from build123d import *

# Parameters (mm, degrees)
SKETCH1_W           = 35.56
SKETCH1_H           = 25.08
BOSS_EXTRUDE1_DEPTH = 0.95
SKETCH2_W           = 26.5
SKETCH2_H           = 18
BOSS_EXTRUDE2_DEPTH = 1.5
BOSS_EXTRUDE3_DEPTH = 1.5
SKETCH4_W           = 10
SKETCH4_H           = 3.18
BOSS_EXTRUDE4_DEPTH = 1.56
SKETCH5_R           = 1
SKETCH5_R_2         = 0.875
SKETCH5_R_3         = 0.2
BOSS_EXTRUDE5_DEPTH = 1.5
SKETCH6_W           = 15.5
SKETCH6_H           = 1.85
SKETCH6_W_2         = 15
SKETCH6_H_2         = 1.35
BOSS_EXTRUDE6_DEPTH = 0.75
SKETCH7_R           = 1
CUT_EXTRUDE1_DEPTH  = 3.51
SKETCH8_R           = 1
CUT_EXTRUDE2_DEPTH  = 3.45
SKETCH9_R           = 1.7
SKETCH9_R_2         = 1
BOSS_EXTRUDE7_DEPTH = 0.0025
SKETCH10_R          = 1.7
SKETCH10_R_2        = 1
BOSS_EXTRUDE8_DEPTH = 0.0025
FILLET1_R           = 0.25
SKETCH11_W          = 2.494146152
SKETCH11_H          = 2.219681882
BOSS_EXTRUDE9_DEPTH = 0.0025


with BuildPart() as part:
    # Sketch1 → Boss-Extrude1 (new body)
    with BuildSketch(Plane(origin=(0, 0, 0), x_dir=(1, 0, 0), z_dir=(0, 1, 0))):
        Rectangle(SKETCH1_W, SKETCH1_H)
    extrude(amount=BOSS_EXTRUDE1_DEPTH)

    # Sketch2 → Boss-Extrude2 (add)
    with BuildSketch(Plane(origin=(0, 0.95, 0), x_dir=(1, 0, 0), z_dir=(0, 1, 0))):
        with Locations((3.68, 2.69)):
            Rectangle(SKETCH2_W, SKETCH2_H)
    extrude(amount=BOSS_EXTRUDE2_DEPTH)

    # Sketch3 → Boss-Extrude3 (add)
    with BuildSketch(Plane.XZ):
        Polygon((16.93, 6.31), (16.93, -11.69), (-11.22, -11.69), (-11.22, -8.69), (-16.47, -8.69), (-16.47, 6.31), align=None)
    extrude(amount=BOSS_EXTRUDE3_DEPTH)

    # Sketch4 → Boss-Extrude4 (add)
    with BuildSketch(Plane(origin=(0, 0.95, 0), x_dir=(1, 0, 0), z_dir=(0, 1, 0))):
        with Locations((-9.78, -10.1)):
            Rectangle(SKETCH4_W, SKETCH4_H)
    extrude(amount=BOSS_EXTRUDE4_DEPTH)

    # Sketch5 → Boss-Extrude5 (add)
    with BuildSketch(Plane(origin=(0, 0.95, 0), x_dir=(1, 0, 0), z_dir=(0, 1, 0))):
        with Locations((-12.78, -2.54)):
            Circle(SKETCH5_R)
        with Locations((-12.78, -2.54)):
            Circle(SKETCH5_R_2, mode=Mode.SUBTRACT)
        with Locations((-12.78, -2.54)):
            Circle(SKETCH5_R_3)
    extrude(amount=BOSS_EXTRUDE5_DEPTH)

    # Sketch6 → Boss-Extrude6 (add)
    with BuildSketch(Plane.XZ):
        with Locations((5.73, 9.315)):
            Rectangle(SKETCH6_W, SKETCH6_H)
        with Locations((5.73, 9.315)):
            Rectangle(SKETCH6_W_2, SKETCH6_H_2, mode=Mode.SUBTRACT)
    extrude(amount=BOSS_EXTRUDE6_DEPTH)

    # Sketch7 → Cut-Extrude1 (cut, through all)
    with BuildSketch(Plane.XZ):
        with Locations((15.96, 9.74)):
            Circle(SKETCH7_R)
    extrude(amount=-CUT_EXTRUDE1_DEPTH, mode=Mode.SUBTRACT)

    # Sketch8 → Cut-Extrude2 (cut, through all)
    with BuildSketch(Plane(origin=(0, 0.95, 0), x_dir=(1, 0, 0), z_dir=(0, 1, 0))):
        with Locations((-12.98, 11.18)):
            Circle(SKETCH8_R)
    extrude(amount=-CUT_EXTRUDE2_DEPTH, mode=Mode.SUBTRACT)

    # Sketch9 → Boss-Extrude7 (add)
    with BuildSketch(Plane(origin=(0, 0.95, 0), x_dir=(1, 0, 0), z_dir=(0, 1, 0))):
        with Locations((15.96, -9.74)):
            Circle(SKETCH9_R)
        with Locations((15.96, -9.74)):
            Circle(SKETCH9_R_2, mode=Mode.SUBTRACT)
        with BuildLine():
            Line((-11.96, 12.54), (-14, 12.54))
            ThreePointArc((-14, 12.54), (-12.98, 9.48), (-11.96, 12.54))
        make_face()
        with Locations((-12.98, 11.18)):
            Circle(SKETCH9_R_2, mode=Mode.SUBTRACT)
    extrude(amount=BOSS_EXTRUDE7_DEPTH)

    # Sketch10 → Boss-Extrude8 (add)
    with BuildSketch(Plane.XZ):
        with Locations((15.96, 9.74)):
            Circle(SKETCH10_R)
        with Locations((15.96, 9.74)):
            Circle(SKETCH10_R_2, mode=Mode.SUBTRACT)
        with BuildLine():
            Line((-11.96, -12.54), (-14, -12.54))
            ThreePointArc((-14, -12.54), (-12.98, -9.48), (-11.96, -12.54))
        make_face()
        with Locations((-12.98, -11.18)):
            Circle(SKETCH10_R_2, mode=Mode.SUBTRACT)
    extrude(amount=BOSS_EXTRUDE8_DEPTH)

    # Fillet1
    fillet1_edges = [part.edges().sort_by_distance(p)[0] for p in [
        (-9.57, 2.45, -2.69),
        (3.68, 2.45, 6.31),
        (16.93, 2.45, -2.69),
        (3.68, 2.45, -11.69),
        (2.855, -1.5, -11.69),
        (16.93, -1.5, -2.69),
        (0.23, -1.5, 6.31),
        (-16.47, -1.5, -1.19),
        (-13.845, -1.5, -8.69),
        (-11.22, -1.5, -10.19),
    ]]
    fillet(fillet1_edges, radius=FILLET1_R)

    # Sketch11 → Boss-Extrude9 (add)
    with BuildSketch(Plane(origin=(0, 0.95, 0), x_dir=(1, 0, 0), z_dir=(0, 1, 0))):
        with Locations((-12.78, -2.54)):
            Rectangle(SKETCH11_W, SKETCH11_H)
    extrude(amount=BOSS_EXTRUDE9_DEPTH)


solid = part.part
For this review, take the finished solid that the model builds, in its own axes (mm). A direction names the side the tool comes from. Round coordinates to 2 decimals unless told otherwise and drop trailing zeros. Order: outer loops, then holes, each group sorted by start corner. A loop starts at its lowest first (then second) coordinate and runs counter-clockwise, first axis right, second up. Notation, with made-up numbers: (44.25, 55.5) -> (92.25, 55.5) arc R21 cw to (92.25, 62.5) -> close; hole circle Ø9 at (-35, -4.5). An arc over 180 degrees is marked (long way). Write item = value, one per line. Start each with the question number.
1) Take a section at B-B on x = 3. State the section outline as (y, z) points.
2) The part is to be moulded in two halves that separate along Z. For faces 5 (the face through (-14.78, 2, 10)), 6 (the face through (-14, -1, -8.69)), 7 (the face through (0, 0, 7)), say which applies: +Z half, -Z half, draft (parallel to the pull), parting line (faces both ways), or undercut.
3) Take a section at D-D on z = 6.75. State the section outline as (x, y) points, plus the area to 3 significant figures.
4) Take a section at C-C on z = -4. State the section outline as (x, y) points.
5) To check wall thickness, follow line 1 (Z direction, x = -1.5, y = -0.15); line 2 (Z direction, x = 16, y = 0.65); line 3 (Z direction, x = -12.98, y = 0.55). State the ranges of each line that lie inside material, in increasing order. Write a range as from..to.
6) Tool access review of faces 1 (the face through (3, 2, 6.31)), 2 (the face through (-11.22, -1, -10)), 3 (the face through (-16.47, -1, -1)), 4 (the face through (3, 2.45, -3)): name each direction out of +Z, -Z, +X, -X, +Y, -Y from which nothing blocks a thin tool from reaching the whole face with its end or side.
7) Insertion check: pin 1 (1.8 mm diameter, centred on x = -13, z = 2.5, fed in from +Y); pin 2 (0.5 mm diameter, centred on y = 1.5, z = 10.5, fed in from -X); pin 3 (1.5 mm diameter, centred on x = 3, y = 2, fed in from -Z). Each pin has a flat end and moves straight along its axis. Give the tip position at first contact, or say it passes through.
Verdict:
q1.outline = (-1.5, -11.44) arc R0.25 ccw to (-1.25, -11.69) -> (0, -11.69) -> (0, -12.54) -> (0.95, -12.54) -> (0.95, -11.69) -> (2.2, -11.69) arc R0.25 ccw to (2.45, -11.44) -> (2.45, 6.06) arc R0.25 ccw to (2.2, 6.31) -> (0.95, 6.31) -> (0.95, 12.54) -> (0, 12.54) -> (0, 10.24) -> (-0.75, 10.24) -> (-0.75, 9.99) -> (0, 9.99) -> (0, 8.64) -> (-0.75, 8.64) -> (-0.75, 8.39) -> (0, 8.39) -> (0, 6.31) -> (-1.25, 6.31) arc R0.25 ccw to (-1.5, 6.06) -> close
q2.face_5 = draft
q2.face_6 = -Z half
q2.face_7 = undercut
q3.outline = (-17.78, 0) -> (17.78, 0) -> (17.78, 0.95) -> (-17.78, 0.95) -> close
q3.area = 33.8 mm2
q4.outline = (-17.78, 0) -> (-16.47, 0) -> (-16.47, -1.25) arc R0.25 ccw to (-16.22, -1.5) -> (16.68, -1.5) arc R0.25 ccw to (16.93, -1.25) -> (16.93, 0) -> (17.78, 0) -> (17.78, 0.95) -> (16.93, 0.95) -> (16.93, 2.2) arc R0.25 ccw to (16.68, 2.45) -> (-9.32, 2.45) arc R0.25 ccw to (-9.57, 2.2) -> (-9.57, 0.95) -> (-17.78, 0.95) -> close
q5.line_1 = -11.69..6.31, 8.39..8.64, 9.99..10.24
q5.line_2 = -12.54..8.74, 10.74..12.54
q5.line_3 = -12.54..-12.18, -10.18..12.54
q6.face_1 = +X, -X, +Y
q6.face_2 = -Z, -X, -Y
q6.face_3 = +Z, -Z, -X, -Y
q6.face_4 = -Z, +X, -X, +Y
q7.pin_1 = 2.45
q7.pin_2 = -14.78
q7.pin_3 = -11.69
